Verification items for the finished model (mm, model axes). A direction names the side the tool comes from. Round coordinates to 2 decimals unless told otherwise and drop trailing zeros. Loops run counter-clockwise (first coordinate to the right, second up) from the corner with the lowest first, then second, coordinate; pieces in that order, holes last. Notation, with made-up numbers: M 9.5,58.5 L 64.5,58.5 A14 cw 64.5,76.5 Z; hole C -38,82.5 d11. An arc over 180 degrees is marked long. One line per item, written item: value.
from build123d import *

# Parameters (mm, degrees)
F0_W     = 23.1
F0_H     = 8
F0_R     = 1.55
F0_H_2   = 3
F1_DEPTH = 2
F2_W     = 23.1
F2_H     = 3
F3_DEPTH = 22


with BuildPart() as f1:
    # F0 (on Top) → F1 (new body)
    with BuildSketch(Plane.XY):
        Rectangle(F0_W, F0_H)
        with Locations((-7, 0)):
            Circle(F0_R, mode=Mode.SUBTRACT)
        with Locations((7, 0)):
            Circle(F0_R, mode=Mode.SUBTRACT)
        with Locations((0, 5.5)):
            Rectangle(F0_W, F0_H_2)
    extrude(amount=F1_DEPTH)

    # F2 (on face) → F3 (join)
    with BuildSketch(Plane(origin=(0, 0, 0), x_dir=(1, 0, 0), z_dir=(0, 0, -1))):
        with Locations((0, -5.5)):
            Rectangle(F2_W, F2_H)
    extrude(amount=F3_DEPTH)


solid = f1.part
(1) Sectioned sample at B-B on y = 0. Enter the section's corners in (x, z), and give its area (3 significant figures).
Completed:
outline: M -11.55,0 L -8.55,0 L -8.55,2 L -11.55,2 Z; M -5.45,0 L 5.45,0 L 5.45,2 L -5.45,2 Z; M 8.55,0 L 11.55,0 L 11.55,2 L 8.55,2 Z
area: 33.8 mm^2
(2) Sectioned sample at D-D on z = -16.25. Enter the section's corners in (x, y).
Completed:
outline: M -11.55,4 L 11.55,4 L 11.55,7 L -11.55,7 Z
(3) Thickness scan on L1, parallel to Y at x = -7, z = 1.15; L2, parallel to Z at x = 4.5, y = -3; L3, parallel to Y at x = -8, z = -18.75. Record the ranges inside material, lowest first. Write a range as from..to.
Completed:
L1: y = -4..-1.55, 1.55..7
L2: z = 0..2
L3: y = 4..7
(4) Sectioned sample at A-A on x = 7. Enter the section's corners in (y, z).
Completed:
outline: M -4,0 L -1.55,0 L -1.55,2 L -4,2 Z; M 1.55,0 L 4,0 L 4,-22 L 7,-22 L 7,2 L 1.55,2 Z
(5) Mould release check, pull along Y, two halves, no side actions. Record for faces 3 (the face through (11.55, 5, -7)), 4 (the face through (0, 7, -10)), 5 (the face through (0, -4, 1)), 6 (the face through (-5.522, 0.466, 0.986)): +Y half, -Y half, draft (parallel to the pull), parting line (faces both ways), or undercut.
Completed:
face 3: draft
face 4: +Y half
face 5: -Y half
face 6: undercut
(6) Depth check by flat-ended pin: pin 1 Ø1.5 at (x, z) = (-1, -6) entering from -Y; pin 2 Ø2.5 at (x, y) = (-1.5, 1) entering from -Z. Enter the tip coordinate at first touch or a pass-through.
Completed:
pin 1: stops at y = 4
pin 2: stops at z = 0
(7) Tool access check on faces 1 (the face through (0, 0, 0)), 2 (the face through (-11.55, 5, -7)). Record the directions out of +Z, -Z, +X, -X, +Y, -Y that give a thin tool (end or side, any length) a straight path to the whole face; none if there is none.
Completed:
face 1: -Z, +X, -X, -Y
face 2: +Z, -Z, -X, +Y, -Y
(8) Sectioned sample at C-C on x = 4.5. Enter the section's corners in (y, z).
Completed:
outline: M -4,0 L 4,0 L 4,-22 L 7,-22 L 7,2 L -4,2 Z
